Geometry: final body of the model. Coordinates: model frame, mm. Face numbers are marked on the shaded views. A direction names the side the tool comes from. Coordinates: 2 decimals unless noted, no trailing zeros. Order: outer loops, then holes, each group sorted by start corner. A loop starts at its lowest first (then second) coordinate and runs counter-clockwise, first axis right, second up. Notation, with made-up numbers: M 13.25,-3 L 70.25,-3 A12 ccw 70.25,5 Z; hole C 24.5,9 d1. An arc over 180 degrees is marked long. Write item = value, one per line.
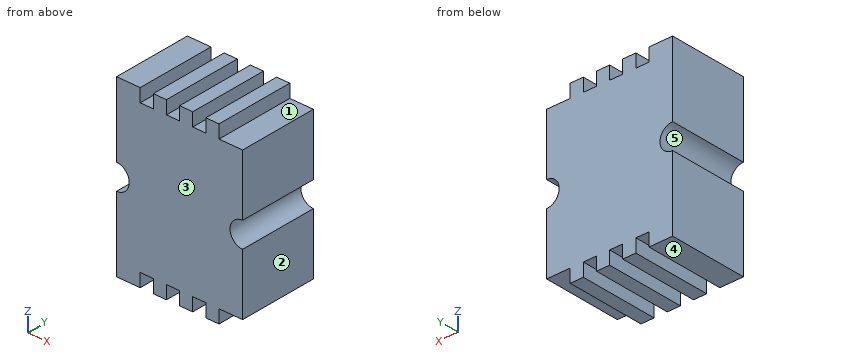
from build123d import *

# Parameters (mm, degrees)
SKETCH1_W           = 40
SKETCH1_H           = 29.4
SKETCH1_R           = 2
BOSS_EXTRUDE1_DEPTH = 20
SKETCH2_W           = 20
SKETCH2_H           = 12.55
CUT_EXTRUDE1_DEPTH  = 3
CUT_EXTRUDE2_REACH  = 42.797
SKETCH2_3_W         = 10
SKETCH2_3_H         = 20
BOSS_EXTRUDE2_REACH = 28.76
SKETCH4_W           = 2.083333333
SKETCH4_H           = 2.1
SKETCH4_W_2         = 2.083333334
SKETCH4_W_3         = 3.75
SKETCH5_W           = 20
SKETCH5_H           = 29.4
CUT_EXTRUDE3_DEPTH  = 7.45


with BuildPart() as part:
    # Sketch1 → Boss-Extrude1 (new body)
    with BuildSketch(Plane(origin=(0, 0, 0), x_dir=(1, 0, 0), z_dir=(0, 1, 0))):
        Rectangle(SKETCH1_W, SKETCH1_H)
        with Locations(Location((-10, 0, 0), (0, 0, 270))):
            Circle(SKETCH1_R, mode=Mode.SUBTRACT)
        with Locations(Location((10, 0, 0), (0, 0, 270))):
            Circle(SKETCH1_R, mode=Mode.SUBTRACT)
    extrude(amount=BOSS_EXTRUDE1_DEPTH)

    # Sketch2 → Cut-Extrude1 (cut)
    with BuildSketch(Plane(origin=(0, 0, -14.7), x_dir=(-1, 0, 0), z_dir=(0, 0, -1))):
        with Locations((0, 13.725)):
            Rectangle(SKETCH2_W, SKETCH2_H)
    cut_extrude1 = extrude(amount=-CUT_EXTRUDE1_DEPTH, mode=Mode.SUBTRACT)

    # Mirror1: Cut-Extrude1 across plane
    add(cut_extrude1.mirror(Plane.XY), mode=Mode.SUBTRACT)

    # Sketch2<3> → Cut-Extrude2 (cut, up to next)
    with BuildSketch(Plane(origin=(0, 0, -14.7), x_dir=(-1, 0, 0), z_dir=(0, 0, -1)), mode=Mode.PRIVATE) as cut_extrude2_sk1:
        with Locations((-15, 10)):
            Rectangle(SKETCH2_3_W, SKETCH2_3_H)
    cut_extrude2_tool1 = extrude(cut_extrude2_sk1.sketch, amount=-CUT_EXTRUDE2_REACH, mode=Mode.PRIVATE) & part.part
    # Sketch2<3> → Cut-Extrude2 (cut, up to next)
    with BuildSketch(Plane(origin=(0, 0, -14.7), x_dir=(-1, 0, 0), z_dir=(0, 0, -1)), mode=Mode.PRIVATE) as cut_extrude2_sk2:
        with Locations((15, 10)):
            Rectangle(SKETCH2_3_W, SKETCH2_3_H)
    cut_extrude2_tool2 = extrude(cut_extrude2_sk2.sketch, amount=-CUT_EXTRUDE2_REACH, mode=Mode.PRIVATE) & part.part
    add(cut_extrude2_tool1.solids().sort_by_distance((15, 10, -14.7))[0], mode=Mode.SUBTRACT)
    add(cut_extrude2_tool2.solids().sort_by_distance((-15, 10, -14.7))[0], mode=Mode.SUBTRACT)

    # Sketch4 → Boss-Extrude2 (add, up to next)
    with BuildSketch(Plane(origin=(0, 20, 0), x_dir=(1, 0, 0), z_dir=(0, 1, 0)), mode=Mode.PRIVATE) as boss_extrude2_sk1:
        with Locations((5.208333334, 12.75)):
            Rectangle(SKETCH4_W, SKETCH4_H)
    boss_extrude2_tool1 = extrude(boss_extrude2_sk1.sketch, amount=-BOSS_EXTRUDE2_REACH, mode=Mode.PRIVATE) - part.part
    # Sketch4 → Boss-Extrude2 (add, up to next)
    with BuildSketch(Plane(origin=(0, 20, 0), x_dir=(1, 0, 0), z_dir=(0, 1, 0)), mode=Mode.PRIVATE) as boss_extrude2_sk2:
        with Locations((1.041666667, 12.75)):
            Rectangle(SKETCH4_W, SKETCH4_H)
    boss_extrude2_tool2 = extrude(boss_extrude2_sk2.sketch, amount=-BOSS_EXTRUDE2_REACH, mode=Mode.PRIVATE) - part.part
    # Sketch4 → Boss-Extrude2 (add, up to next)
    with BuildSketch(Plane(origin=(0, 20, 0), x_dir=(1, 0, 0), z_dir=(0, 1, 0)), mode=Mode.PRIVATE) as boss_extrude2_sk3:
        with Locations((-3.125, 12.75)):
            Rectangle(SKETCH4_W_2, SKETCH4_H)
    boss_extrude2_tool3 = extrude(boss_extrude2_sk3.sketch, amount=-BOSS_EXTRUDE2_REACH, mode=Mode.PRIVATE) - part.part
    # Sketch4 → Boss-Extrude2 (add, up to next)
    with BuildSketch(Plane(origin=(0, 20, 0), x_dir=(1, 0, 0), z_dir=(0, 1, 0)), mode=Mode.PRIVATE) as boss_extrude2_sk4:
        with Locations((-8.125, 12.75)):
            Rectangle(SKETCH4_W_3, SKETCH4_H)
    boss_extrude2_tool4 = extrude(boss_extrude2_sk4.sketch, amount=-BOSS_EXTRUDE2_REACH, mode=Mode.PRIVATE) - part.part
    boss_extrude2_1 = boss_extrude2_tool1.solids().sort_by_distance((5.208333, 20, -12.75))[0]
    add(boss_extrude2_1)
    boss_extrude2_2 = boss_extrude2_tool2.solids().sort_by_distance((1.041667, 20, -12.75))[0]
    add(boss_extrude2_2)
    boss_extrude2_3 = boss_extrude2_tool3.solids().sort_by_distance((-3.125, 20, -12.75))[0]
    add(boss_extrude2_3)
    boss_extrude2_4 = boss_extrude2_tool4.solids().sort_by_distance((-8.125, 20, -12.75))[0]
    add(boss_extrude2_4)
    boss_extrude2 = boss_extrude2_1 + boss_extrude2_2 + boss_extrude2_3 + boss_extrude2_4  # Boss-Extrude2 as one shape, for the pattern or mirror that repeats it

    # Mirror2: Boss-Extrude2 across plane
    add(boss_extrude2.mirror(Plane.XY))

    # Sketch5 → Cut-Extrude3 (cut)
    with BuildSketch(Plane.XZ):
        Rectangle(SKETCH5_W, SKETCH5_H)
    extrude(amount=-CUT_EXTRUDE3_DEPTH, mode=Mode.SUBTRACT)


solid = part.part
1) Mould query, pull axis Z, two halves, no side actions, for the marked faces 3, 4 and 5. Classes: pulls with the +Z half, pulls with the -Z half, needs draft (parallel to the pull), parting line crosses it, or undercut.
Numbers:
face_3 = needs draft
face_4 = pulls with the -Z half
face_5 = undercut
2) Section C-C, the plane x = -5. Return loops of the section in (y, z), and give its area (3 significant figures).
Numbers:
outline = M 7.45,-11.7 L 20,-11.7 L 20,11.7 L 7.45,11.7 Z
area = 294 mm²
3) Pin query (flat end, axial travel): pin 1 (1.5 mm diameter, centred on x = -1, y = 16, fed in from +Z); pin 2 (0.6 mm diameter, centred on y = 14, z = 13.5, fed in from +X); pin 3 (1.9 mm diameter, centred on x = 9, y = 16.5, fed in from -Z). Return the tip coordinate at first contact, or that it passes through.
Numbers:
pin_1 = 11.7
pin_2 = 6.25
pin_3 = -11.7
4) Section A-A, the plane x = 8.5. Return loops of the section in (y, z).
Numbers:
outline = M 7.45,-11.7 L 20,-11.7 L 20,-1.32 L 7.45,-1.32 Z; M 7.45,1.32 L 20,1.32 L 20,11.7 L 7.45,11.7 Z
5) Section B-B, the plane z = 0. Return loops of the section in (x, y).
Numbers:
outline = M -8,7.45 L 8,7.45 L 8,20 L -8,20 Z
6) Set-up query: the marked faces 1 and 2. Return all of +Z, -Z, +X, -X, +Y, -Y with unobstructed straight access to the full face (end or side cutting, diameter ignored); none if empty.
Numbers:
face_1 = +Z, +X, +Y, -Y
face_2 = +Z, -Z, +X, +Y, -Y
7) Line query: L1, parallel to X at y = 14, z = 12.75; L2, parallel to Z at x = 9, y = 17.5; L3, parallel to X at y = 12.5, z = 0. Output: solid intervals per line, ascending.
Numbers:
L1 = -10 to -6.25, -4.17 to -2.08, 0 to 2.08, 4.17 to 6.25
L2 = -11.7 to -1.73, 1.73 to 11.7
L3 = -8 to 8
